from build123d import *

# Parameters (mm, degrees)
F1_DEPTH = 2
F2_DEPTH = 4
F0_W     = 70.7484384206
F0_H     = 2.5396057816
F3_DEPTH = 10
F0_W_2   = 3.0519364719
F4_DEPTH = 10
F6_DEPTH = 2


with BuildPart() as f1:
    # F0 (on Top) → F1 (new body)
    with BuildSketch(Plane.XY):
        Polygon((-33.9991840492, 35.2650536744), (-9.306327631, 0), (12.0563979532, 0), (36.7492543714, 35.2650536744), align=None)
    extrude(amount=F1_DEPTH)

    # F0 (on Top) → F2 (join)
    with BuildSketch(Plane.XY):
        Polygon((-37.0511205211, 35.2650536744), (-12.3582641029, 0), (-9.306327631, 0), (-33.9991840492, 35.2650536744), align=None)
        Polygon((36.7492543714, 35.2650536744), (12.0563979532, 0), (15.1083344251, 0), (39.8011908433, 35.2650536744), align=None)
    extrude(amount=F2_DEPTH)



with BuildPart() as f3:
    # F0 (on Top) → F3 (new body)
    with BuildSketch(Plane.XY):
        with Locations((1.3750351611, 36.5348565652)):
            Rectangle(F0_W, F0_H)
    extrude(amount=F3_DEPTH)


with BuildPart() as f1_1:
    add(f1.part)

    add(f3.part)  # F4 merges F3
    # F0 (on Top) → F4 (join)
    with BuildSketch(Plane.XY):
        with Locations((38.2752226073, 36.5348565652)):
            Rectangle(F0_W_2, F0_H)
        with Locations((-35.5251522851, 36.5348565652)):
            Rectangle(F0_W_2, F0_H)
    extrude(amount=F4_DEPTH)

    # F5 (on face) → F6 (join)
    with BuildSketch(Plane(origin=(10.1378445653, -7.0985951858, 0), x_dir=(0.5735764364, 0.8191520443, 0), z_dir=(0.8191520443, -0.5735764364, 0))):
        Polygon((51.7171509564, 10.0024873391), (8.6657846187, 4), (51.7164660158, 4), align=None)
    extrude(amount=-F6_DEPTH)


solid = f1_1.part
CAD build for the part. Positions are in the model's coordinates, mm. A direction names the side the tool comes from. Give positions to 0.01 mm unless a question says otherwise; leave off trailing zeros. Loops run counter-clockwise (first coordinate to the right, second up) from the corner with the lowest first, then second, coordinate; pieces in that order, holes last. Notation, with made-up numbers: M 87,19.5 L 94,19.5 A17 cw 94,52.5 Z; hole C 30.25,-21.5 d3. An arc over 180 degrees is marked long. One line per question, with ' | ' between items. Start each with the question number.
1. Two-plate mould, pull along Y, no slides. Class faces 6 (the face through (-24.88, 17.88, 1.97)), 7 (the face through (26.5, 20.3, 4)), 8 (the face through (-37.051, 37, 5)), 9 (the face through (24.576, 17.879, 2.986)): pulls with the +Y half, pulls with the -Y half, needs draft (parallel to the pull), parting line crosses it, or undercut.
2. Saw through at B-B on y = 13. Give the cut face in (x, z), plus the area to 3 significant figures.
3. Saw through at C-C on x = -20. Give the cut face in (y, z), plus the area to 3 significant figures.
4. Flat gauge pins, fed straight in: pin 1 (17.5 mm diameter, centred on x = -13.5, y = 25.5, fed in from +Z); pin 2 (5 mm diameter, centred on y = 21, z = 4.5, fed in from +X); pin 3 (8.5 mm diameter, centred on x = -24, y = 22.5, fed in from +Z). Where does each tip first touch, or does it go through?
5. Probe L1, parallel to Y at x = 6, z = 5; L2, parallel to Z at x = -17.5, y = 26; L3, parallel to Z at x = 6, y = 36. List the from-to ranges inside material, lowest first. Write a range as from..to.
6. 3-axis set-ups, long thin cutter, end or side, ignore diameter. For faces 1 (the face through (1, 23, 0)), 2 (the face through (1, 37, 10)), 3 (the face through (1, 22, 2)), 4 (the face through (30.556, 25.549, 5.654)), 5 (the face through (-23, 18, 4)): which of +Z, -Z, +X, -X, +Y, -Y reach the whole face in a straight line?
7. Saw through at A-A on z = 2.75. Give the cut face in (x, y), plus the area to 3 significant figures.
Result sheet:
1) face 6: pulls with the -Y half | face 7: undercut | face 8: needs draft | face 9: undercut
2) outline: M -21.46,0 L 24.21,0 L 24.21,6.21 L 21.77,6.02 L 21.77,4 L 21.16,4 L 21.16,2 L -18.41,2 L -18.41,4 L -21.46,4 Z | area: 109 mm^2
3) outline: M 10.91,0 L 37.8,0 L 37.8,10 L 35.27,10 L 35.27,2 L 15.27,2 L 15.27,4 L 10.91,4 Z | area: 82.8 mm^2
4) pin 1: stops at z = 2 | pin 2: stops at x = 31.56 | pin 3: stops at z = 4
5) L1: y = 35.27..37.8 | L2: z = 0..2 | L3: z = 0..10
6) face 1: -Z, +X, -X, +Y, -Y | face 2: +Z, +X, -X, +Y, -Y | face 3: +Z | face 4: +Z, -X | face 5: +Z, -X, -Y
7) outline: M -37.05,35.27 L -12.36,0 L -9.31,0 L -34,35.27 L 36.75,35.27 L 12.06,0 L 15.11,0 L 39.8,35.27 L 39.8,37.8 L -37.05,37.8 Z | area: 410 mm^2
